The model under review builds one solid part; all positions refer to its coordinate system, in mm. A direction names the side the tool comes from. Give positions to 0.01 mm unless a question says otherwise; leave off trailing zeros. Order: outer loops, then holes, each group sorted by start corner. A loop starts at its lowest first (then second) coordinate and runs counter-clockwise, first axis right, second up. Notation, with made-up numbers: (-37.5, 18) - (19.5, 18) arc R6 cw to (19.5, 28) - close; hole circle Ø4 at (71, -36). An arc over 180 degrees is marked (long way). Use CSV: the item, a comma, the result in double quotes.
```python
from build123d import *

# Parameters (mm, degrees)
EXTRUDE_THIN1_DEPTH = 20
FILLET1_R           = 3
FILLET3_R           = 2
SKETCH3_R           = 2.5
CUT_EXTRUDE1_DEPTH  = 10
SKETCH4_R           = 2.5
CUT_EXTRUDE2_DEPTH  = 10


with BuildPart() as part:
    # Sketch1 → Extrude-Thin1 (new body)
    with BuildSketch(Plane.XY):
        Polygon((0, 0), (0, -20), (20, -20), (20, -21), (-1, -21), (-1, 0), align=None)
    extrude(amount=EXTRUDE_THIN1_DEPTH)

    # Fillet1
    fillet1_edges = [part.edges().sort_by_distance(p)[0] for p in [
        (-1, -21, 10),
    ]]
    fillet(fillet1_edges, radius=FILLET1_R)

    # Fillet3
    fillet3_edges = [part.edges().sort_by_distance(p)[0] for p in [
        (0, -20, 10),
    ]]
    fillet(fillet3_edges, radius=FILLET3_R)

    # Sketch3 → Cut-Extrude1 (cut)
    with BuildSketch(Plane(origin=(0, 0, 0), x_dir=(0, 0, -1), z_dir=(1, 0, 0))):
        with Locations(Location((-10, -9, 0), (0, 0, 90))):
            Circle(SKETCH3_R)
    extrude(amount=-CUT_EXTRUDE1_DEPTH, mode=Mode.SUBTRACT)

    # Sketch4 → Cut-Extrude2 (cut)
    with BuildSketch(Plane(origin=(0, -20, 0), x_dir=(1, 0, 0), z_dir=(0, 1, 0))):
        with Locations(Location((11, -10, 0), (0, 0, 270))):
            Circle(SKETCH4_R)
    extrude(amount=-CUT_EXTRUDE2_DEPTH, mode=Mode.SUBTRACT)


solid = part.part
```
Item 1: Take a section at A-A, the plane x = 11. Give the boundary of the cut face in (y, z).
Results list:
outline,"(-21, 0) - (-20, 0) - (-20, 7.5) - (-21, 7.5) - close; (-21, 12.5) - (-20, 12.5) - (-20, 20) - (-21, 20) - close"
Item 2: Wall thickness on L1, parallel to Z at x = -0.65, y = -9; L2, parallel to X at y = -12.5, z = 13.75; L3, parallel to Y at x = 12.5, z = 5.25: over which ranges is each line inside the solid? List them lowest first.
Results list:
L1,"z = 0 to 7.5, 12.5 to 20"
L2,"x = -1 to 0"
L3,"y = -21 to -20"
Item 3: Take a section at C-C, the plane z = 10. Give the boundary of the cut face in (x, y).
Results list:
outline,"(-1, -18) arc R3 ccw to (2, -21) - (8.5, -21) - (8.5, -20) - (2, -20) arc R2 cw to (0, -18) - (0, -11.5) - (-1, -11.5) - close; (-1, -6.5) - (0, -6.5) - (0, 0) - (-1, 0) - close; (13.5, -21) - (20, -21) - (20, -20) - (13.5, -20) - close"
Item 4: Mouldability with a two-part tool opening along X and no side actions: class faces 3 (the face through (8.56, -20.49, 9.46)), 4 (the face through (-0.49, -9.54, 7.56)), 5 (the face through (0, -11, 8)) as pulls with the +X half, pulls with the -X half, needs draft (parallel to the pull), parting line crosses it, or undercut.
Results list:
face 3,"undercut"
face 4,"needs draft"
face 5,"pulls with the +X half"
Item 5: Take a section at B-B, the plane y = -9. Give the boundary of the cut face in (x, z), and give its area (3 significant figures).
Results list:
outline,"(-1, 0) - (0, 0) - (0, 7.5) - (-1, 7.5) - close; (-1, 12.5) - (0, 12.5) - (0, 20) - (-1, 20) - close"
area,"15.0 mm2"
Item 6: Clearance check with flat-ended pins moving along their axes: pin 1 (12 mm diameter, centred on x = 2.5, y = -18.5, fed in from -Z); pin 2 (5.5 mm diameter, centred on y = -11, z = 9.5, fed in from +X); pin 3 (4 mm diameter, centred on x = 7, z = 14.5, fed in from +Y). State where each tip first meets the part, or that it passes through.
Results list:
pin 1,"stops at z = 0"
pin 2,"stops at x = 0"
pin 3,"stops at y = -20"
Item 7: Tool access review of faces 1 (the face through (-0.1, -20.14, 10.14)), 2 (the face through (13, -20, 8)): name each direction out of +Z, -Z, +X, -X, +Y, -Y from which nothing blocks a thin tool from reaching the whole face with its end or side.
Results list:
face 1,"+Z, -Z, -X, -Y"
face 2,"+Z, -Z, +X, +Y"
Item 8: Take a section at D-D, the plane z = 16.75. Give the boundary of the cut face in (x, y), and give its area (3 significant figures).
Results list:
outline,"(-1, -18) arc R3 ccw to (2, -21) - (20, -21) - (20, -20) - (2, -20) arc R2 cw to (0, -18) - (0, 0) - (-1, 0) - close"
area,"39.9 mm2"
